For this review, take the finished solid that the model builds, in its own axes (mm). Coordinates: 2 decimals unless noted, no trailing zeros. Loops run counter-clockwise (first coordinate to the right, second up) from the corner with the lowest first, then second, coordinate; pieces in that order, holes last. Notation, with made-up numbers: (16, -5.75) -> (31, -5.75) arc R24 ccw to (31, 22.25) -> close; hole circle Ø4 at (59.5, 62.25). An arc over 180 degrees is marked (long way). Answer in a Markdown table with one row per item.
Autodesk Inventor part; units mm, degrees
ref_plane "YZ Plane" through (0, 0, 0) normal (1, 0, 0) x (0, 1, 0)
ref_plane "XZ Plane" through (0, 0, 0) normal (0, 1, 0) x (-1, 0, 0)
ref_plane "XY Plane" through (0, 0, 0) normal (0, 0, 1) x (1, 0, 0)
sketch "Sketch1" plane through (0, 0, 0) normal (0, 0, 1) x (1, 0, 0)
  line L0 (0, 0) -> (0, 4438.8737)
  line L1 (0, 4438.8737) -> (100, 4438.8737)
  line L2 (100, 4438.8737) -> (200, 0)
  line L3 (200, 0) -> (0, 0)
  circle A0 centre (0, 0) radius 30
  line L4 (0, 1479.6246) -> (166.6667, 1479.6246)
  line L5 (0, 2959.2492) -> (133.3333, 2959.2492)
  circle A1 centre (0, 1479.6246) radius 30
  circle A2 centre (0, 2959.2492) radius 30
  line L6 (190.8761, 405) -> (120.8761, 405)
  line L7 (120.8761, 405) -> (120.8761, 410)
  line L8 (120.8761, 410) -> (190.8761, 410)
  line L9 (190.8761, 410) -> (190.8761, 405)
  line L10 (109.6148, 909.8732) -> (179.6148, 909.8732)
  line L11 (179.6148, 904.8732) -> (109.6148, 904.8732)
  line L12 (109.6148, 904.8732) -> (109.6148, 909.8732)
  line L13 (179.6148, 909.8732) -> (179.6148, 904.8732)
  line L14 (98.3535, 1409.7463) -> (168.3535, 1409.7463)
  line L15 (168.3535, 1404.7463) -> (98.3535, 1404.7463)
  line L16 (98.3535, 1404.7463) -> (98.3535, 1409.7463)
  line L17 (168.3535, 1409.7463) -> (168.3535, 1404.7463)
  line L18 (87.0923, 1909.6195) -> (157.0923, 1909.6195)
  line L19 (157.0923, 1904.6195) -> (87.0923, 1904.6195)
  line L20 (87.0923, 1904.6195) -> (87.0923, 1909.6195)
  line L21 (157.0923, 1909.6195) -> (157.0923, 1904.6195)
  line L22 (75.831, 2409.4927) -> (145.831, 2409.4927)
  line L23 (145.831, 2404.4927) -> (75.831, 2404.4927)
  line L24 (75.831, 2404.4927) -> (75.831, 2409.4927)
  line L25 (145.831, 2409.4927) -> (145.831, 2404.4927)
  line L26 (64.5698, 2909.3658) -> (134.5698, 2909.3658)
  line L27 (134.5698, 2904.3658) -> (64.5698, 2904.3658)
  line L28 (64.5698, 2904.3658) -> (64.5698, 2909.3658)
  line L29 (134.5698, 2909.3658) -> (134.5698, 2904.3658)
  line L30 (53.3085, 3409.239) -> (123.3085, 3409.239)
  line L31 (123.3085, 3404.239) -> (53.3085, 3404.239)
  line L32 (53.3085, 3404.239) -> (53.3085, 3409.239)
  line L33 (123.3085, 3409.239) -> (123.3085, 3404.239)
  line L34 (42.0472, 3909.1122) -> (112.0472, 3909.1122)
  line L35 (112.0472, 3904.1122) -> (42.0472, 3904.1122)
  line L36 (42.0472, 3904.1122) -> (42.0472, 3909.1122)
  line L37 (112.0472, 3909.1122) -> (112.0472, 3904.1122)
  line L38 (0, 1629.6246) -> (163.2874, 1629.6246)
  line L39 (0, 3079.2492) -> (130.6299, 3079.2492)
  circle A3 centre (20, 3059.2492) radius 9
  circle A4 centre (117.3833, 2779.2492) radius 9
  circle A5 centre (139.9031, 1779.6246) radius 9
  line L40 (139.9031, 1779.6246) -> (117.3833, 2779.2492)
  point P0 (30, 2959.2492)
  point P1 (0, 2929.2492)
  point P2 (0, 1509.6246)
  point P3 (0, 1449.6246)
  point P4 (0, 30)
  point P5 (30, 0)
  point P6 (190.7634, 410)
  point P7 (179.5022, 909.8732)
  point P8 (168.3535, 1404.7463)
  point P9 (168.2409, 1409.7463)
  point P10 (30, 1479.6246)
  point P11 (157.0923, 1904.6195)
  point P12 (156.9796, 1909.6195)
  point P13 (145.831, 2404.4927)
  point P14 (145.7184, 2409.4927)
  point P15 (134.5698, 2904.3658)
  point P16 (134.4571, 2909.3658)
  point P17 (0, 2989.2492)
  dimension "d65" = 100
  dimension "d67" = 200
  dimension "d68" = 60
  dimension "d69" = 1480
  dimension "d70" = 1480
  dimension "d71" = 1480
  dimension "d72" = 5
  dimension "d73" = 70
  dimension "d74" = 410
  dimension "d77" = 500
  dimension "d82" = 120
  dimension "d83" = 150
  dimension "d88" = 18
  dimension "d89" = 20
  dimension "d90" = 20
  dimension "d91" = 20
  dimension "d92" = 300
  dimension "d93" = 300
extrude "Plate3" add sketch "Sketch1" along normal blind 4 contours L39 L2 L5 A2 L0 | L5 L2 L26 L28 L27 L22 L24 L23 L40 L18 L20 L19 L38 L0 A2 | L38 L2 L4 A1 L0 | L18 L40 L23 L2
chamfer "Corner Chamfer2" distance 3 angle 45 6 edges at (157.0923, 1904.6195, 2) (156.9796, 1909.6195, 2) (145.831, 2404.4927, 2) (145.7184, 2409.4927, 2) (134.5698, 2904.3658, 2) (134.4571, 2909.3658, 2)
equation "\"BendRadius\" = Thickness"
equation "\"BendReliefWidth\" = Thickness"
equation "\"BendReliefDepth\" = 0.5 * Thickness"
equation "\"CornerReliefSize\" = 4 * Thickness"
equation "\"MinimumRemnant\" = 2 * Thickness"
equation "\"TransitionRadius\" = BendRadius"
equation "\"JacobiRadiusSize\" = BendRadius"
equation "\"GapSize\" = Thickness"
properties part number "GBK 3212 central second rib" material "Steel"
Item 1: Take a section at C-C, the plane y = 2496. State the section outline as (x, z) points, and give its area (3 significant figures).
Worked answers:
| item | result |
|---|---|
| outline | (0, 0) -> (143.77, 0) -> (143.77, 4) -> (0, 4) -> close |
| area | 575 mm² |
Item 2: For L1, parallel to Y at x = 97, z = 1.5; L2, parallel to Y at x = 117, z = 1.55; L3, parallel to X at y = 2533.5, z = 2.1, list the stretches that pass through material, from the lowest coordinate up.
Worked answers:
| item | result |
|---|---|
| L1 | 1479.62 to 1904.62, 1909.62 to 2404.49, 2409.49 to 2904.37, 2909.37 to 3079.25 |
| L2 | 1479.62 to 1904.62, 1909.62 to 2404.49, 2409.49 to 2770.26, 2788.24 to 2904.37, 2909.37 to 3079.25 |
| L3 | 0 to 142.92 |
Item 3: The part is to be moulded in two halves that separate along Y. For faces 1 (the cylindrical face through (20.98, 1501.07, 1.97)), 2 (the cylindrical face through (29.993, 2959.909, 1.972)), 3 (the flat face through (82, 2291, 4)), say which applies: +Y half, -Y half, draft (parallel to the pull), parting line (faces both ways), or undercut.
Worked answers:
| item | result |
|---|---|
| face 1 | -Y half |
| face 2 | undercut |
| face 3 | draft |
Item 4: Insertion check: pin 1 (1.5 mm diameter, centred on x = 110, y = 2478.5, fed in from -Z); pin 2 (1.2 mm diameter, centred on y = 2408, z = 2.5, fed in from +X). Each pin has a flat end and moves straight along its axis. Give the tip position at first contact, or say it passes through.
Worked answers:
| item | result |
|---|---|
| pin 1 | z = 0 |
| pin 2 | x = 75.83 |
Item 5: Take a section at A-A, the plane z = 0.65. State the section outline as (x, y) points.
Worked answers:
| item | result |
|---|---|
| outline | (0, 1509.62) arc R30 cw to (30, 1479.62) -> (166.67, 1479.62) -> (157.16, 1901.62) -> (154.09, 1904.62) -> (87.09, 1904.62) -> (87.09, 1909.62) -> (153.98, 1909.62) -> (156.91, 1912.62) -> (145.9, 2401.49) -> (142.83, 2404.49) -> (75.83, 2404.49) -> (75.83, 2409.49) -> (142.72, 2409.49) -> (145.65, 2412.49) -> (134.64, 2901.37) -> (131.57, 2904.37) -> (64.57, 2904.37) -> (64.57, 2909.37) -> (131.46, 2909.37) -> (134.39, 2912.37) -> (130.63, 3079.25) -> (0, 3079.25) -> (0, 2989.25) arc R30 cw to (0, 2929.25) -> close; hole circle Ø18 at (20, 3059.25); hole circle Ø18 at (117.38, 2779.25); hole circle Ø18 at (139.9, 1779.62) |
Item 6: Take a section at B-B, the plane y = 2016. State the section outline as (x, z) points, and give its area (3 significant figures).
Worked answers:
| item | result |
|---|---|
| outline | (0, 0) -> (154.58, 0) -> (154.58, 4) -> (0, 4) -> close |
| area | 618 mm² |
